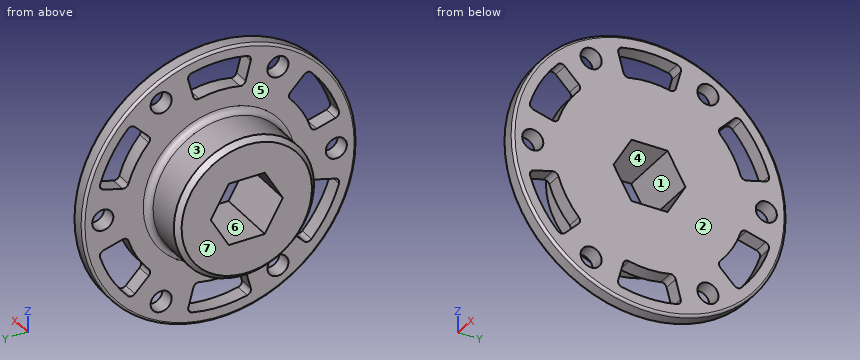
from build123d import *

# Parameters (mm, degrees)
SKETCH1_W                      = 3.175
SKETCH1_H                      = 27.94
CUT_EXTRUDE1_DEPTH             = 4.175
CUT_EXTRUDE2_DEPTH             = 4.175
CUT_EXTRUDE3_DEPTH             = 4.175
CUT_EXTRUDE4_DEPTH             = 4.175
CUT_EXTRUDE5_DEPTH             = 4.175
CUT_EXTRUDE6_DEPTH             = 4.175
SKETCH8_R                      = 14.294919975
BOSS_EXTRUDE1_DEPTH            = 9.525
CUT_EXTRUDE7_DEPTH             = 13.7
F_4_3_4_3_DIAMETER_HOLE1_D     = 4.3
F_4_3_4_3_DIAMETER_HOLE1_DEPTH = 12.7
CHAMFER1_SIZE                  = 1
FILLET1_R                      = 0.5
FILLET2_R                      = 1
FILLET3_R                      = 1.27


with BuildPart() as part:
    # Sketch1 → Revolve1 (revolve)
    with BuildSketch(Plane(origin=(0, 0, 0), x_dir=(-1, 0, 0), z_dir=(0, 0, -1))):
        with Locations((-11.1125, 13.97)):
            Rectangle(SKETCH1_W, SKETCH1_H)
    revolve(axis=Axis((12.7, 0, 0), (-1, 0, 0)))

    # Sketch2 → Cut-Extrude1 (cut, through all)
    with BuildSketch(Plane.ZY.offset(-9.525)):
        with BuildLine():
            Line((-13.806531048, -13.770610024), (-18.049174487, -18.013253463))
            ThreePointArc((-18.049174487, -18.013253463), (-12.738999884, -22.089995065), (-6.550803522, -24.644207701))
            Line((-6.550803522, -24.644207701), (-4.997885221, -18.848637704))
            ThreePointArc((-4.997885221, -18.848637704), (-9.738999389, -16.893841804), (-13.806531048, -13.770610024))
        make_face()
    extrude(amount=-CUT_EXTRUDE1_DEPTH, mode=Mode.SUBTRACT)

    # Sketch3 → Cut-Extrude2 (cut, through all)
    with BuildSketch(Plane.ZY.offset(-9.525)):
        with BuildLine():
            Line((5.022432582, -18.842111637), (6.57534786, -24.637670355))
            ThreePointArc((6.57534786, -24.637670355), (12.760996954, -22.077295051), (18.067108165, -17.995266116))
            Line((18.067108165, -17.995266116), (13.824456468, -13.752614419))
            ThreePointArc((13.824456468, -13.752614419), (9.760996476, -16.88114178), (5.022432582, -18.842111637))
        make_face()
    extrude(amount=-CUT_EXTRUDE2_DEPTH, mode=Mode.SUBTRACT)

    # Sketch4 → Cut-Extrude3 (cut, through all)
    with BuildSketch(Plane.ZY.offset(-9.525)):
        with BuildLine():
            Line((18.82896363, -5.071501614), (24.624522347, -6.624416892))
            ThreePointArc((24.624522347, -6.624416892), (25.499996837, 0.012700014), (24.617911686, 6.648941586))
            Line((24.617911686, 6.648941586), (18.822341689, 5.096023285))
            ThreePointArc((18.822341689, 5.096023285), (19.499995864, 0.012700024), (18.82896363, -5.071501614))
        make_face()
    extrude(amount=-CUT_EXTRUDE3_DEPTH, mode=Mode.SUBTRACT)

    # Sketch5 → Cut-Extrude4 (cut, through all)
    with BuildSketch(Plane.ZY.offset(-9.525)):
        with BuildLine():
            Line((13.806531048, 13.770610024), (18.049174487, 18.013253463))
            ThreePointArc((18.049174487, 18.013253463), (12.738999884, 22.089995065), (6.550803522, 24.644207701))
            Line((6.550803522, 24.644207701), (4.997885221, 18.848637704))
            ThreePointArc((4.997885221, 18.848637704), (9.738999389, 16.893841804), (13.806531048, 13.770610024))
        make_face()
    extrude(amount=-CUT_EXTRUDE4_DEPTH, mode=Mode.SUBTRACT)

    # Sketch6 → Cut-Extrude5 (cut, through all)
    with BuildSketch(Plane.ZY.offset(-9.525)):
        with BuildLine():
            Line((-24.617911686, -6.648941586), (-18.822341689, -5.096023285))
            ThreePointArc((-18.822341689, -5.096023285), (-19.499995864, -0.012700024), (-18.82896363, 5.071501614))
            Line((-18.82896363, 5.071501614), (-24.624522347, 6.624416892))
            ThreePointArc((-24.624522347, 6.624416892), (-25.499996837, -0.012700014), (-24.617911686, -6.648941586))
        make_face()
    extrude(amount=-CUT_EXTRUDE5_DEPTH, mode=Mode.SUBTRACT)

    # Sketch7 → Cut-Extrude6 (cut, through all)
    with BuildSketch(Plane(origin=(12.7, 0, 0), x_dir=(0, 0, -1), z_dir=(1, 0, 0))):
        with BuildLine():
            Line((6.57534786, 24.637670355), (5.022432582, 18.842111637))
            ThreePointArc((5.022432582, 18.842111637), (9.760996476, 16.88114178), (13.824456468, 13.752614419))
            Line((13.824456468, 13.752614419), (18.067108165, 17.995266116))
            ThreePointArc((18.067108165, 17.995266116), (12.760996954, 22.077295051), (6.57534786, 24.637670355))
        make_face()
    extrude(amount=-CUT_EXTRUDE6_DEPTH, mode=Mode.SUBTRACT)

    # Sketch8 → Boss-Extrude1 (add)
    with BuildSketch(Plane.ZY.offset(-9.525)):
        Circle(SKETCH8_R)
    extrude(amount=BOSS_EXTRUDE1_DEPTH)

    # Sketch9 → Cut-Extrude7 (cut, through all)
    with BuildSketch(Plane(origin=(12.7, 0, 0), x_dir=(0, 0, -1), z_dir=(1, 0, 0))):
        Polygon((-6.3627, 3.673506558), (-6.3627, -3.673506558), (0, -7.347013116), (6.3627, -3.673506558), (6.3627, 3.673506558), (0, 7.347013116), align=None)
    extrude(amount=-CUT_EXTRUDE7_DEPTH, mode=Mode.SUBTRACT)

    # Ø4.3 (4.3) Diameter Hole1
    with Locations(Plane(origin=(12.7, 0, 0), x_dir=(0, 0, -1), z_dir=(1, 0, 0))):
        with Locations((20.622229928, 11.90625), (20.622229928, -11.90625), (0, -23.8125), (-20.622229928, -11.90625), (-20.622229928, 11.90625), (0, 23.8125)):
            Hole(F_4_3_4_3_DIAMETER_HOLE1_D / 2, depth=F_4_3_4_3_DIAMETER_HOLE1_DEPTH)

    # Chamfer1
    chamfer1_edges = [part.edges().sort_by_distance(p)[0] for p in [
        (0, 0, -14.294919975),
    ]]
    chamfer(chamfer1_edges, length=CHAMFER1_SIZE)

    # Fillet1
    fillet1_edges = [part.edges().sort_by_distance(p)[0] for p in [
        (9.525, -27.94, 0),
        (12.7, -27.94, 0),
    ]]
    fillet(fillet1_edges, radius=FILLET1_R)

    # Fillet2
    fillet2_edges = [part.edges().sort_by_distance(p)[0] for p in [
        (11.1125, -13.770610024, -13.806531048),
        (11.1125, -18.848637704, -4.997885221),
        (11.1125, -24.644207701, -6.550803522),
        (11.1125, -18.013253463, -18.049174487),
        (11.1125, -18.842111637, 5.022432582),
        (11.1125, -13.752614419, 13.824456468),
        (11.1125, -17.995266116, 18.067108165),
        (11.1125, -24.637670355, 6.57534786),
        (11.1125, -5.071501614, 18.82896363),
        (11.1125, 5.096023285, 18.822341689),
        (11.1125, 6.648941586, 24.617911686),
        (11.1125, -6.624416892, 24.624522347),
        (11.1125, 13.770610024, 13.806531048),
        (11.1125, 18.848637704, 4.997885221),
        (11.1125, 24.644207701, 6.550803522),
        (11.1125, 18.013253463, 18.049174487),
        (11.1125, -6.648941586, -24.617911686),
        (11.1125, 6.624416892, -24.624522347),
        (11.1125, 5.071501614, -18.82896363),
        (11.1125, -5.096023285, -18.822341689),
        (11.1125, 24.637670355, -6.57534786),
        (11.1125, 17.995266116, -18.067108165),
        (11.1125, 13.752614419, -13.824456468),
        (11.1125, 18.842111637, -5.022432582),
    ]]
    fillet(fillet2_edges, radius=FILLET2_R)

    # Fillet3
    fillet3_edges = [part.edges().sort_by_distance(p)[0] for p in [
        (9.525, 0, -14.294919975),
    ]]
    fillet(fillet3_edges, radius=FILLET3_R)


solid = part.part
The model under review builds one solid part; all positions refer to its coordinate system, in mm. Face numbers are marked on the shaded views. A direction names the side the tool comes from. Give positions to 0.01 mm unless a question says otherwise; leave off trailing zeros. Write each loop counter-clockwise with the first axis right and the second up, starting at its lowest first coordinate (ties: lowest second). Pieces come first, ordered by that corner, then holes.
1. Wall thickness on L1, parallel to Y at x = 11.25, z = 0; L2, parallel to Z at x = 10.5, y = 21; L3, parallel to Y at x = 4.5, z = -13: over which ranges is each line inside the solid? List them lowest first.
2. Add section B-B, the plane x = 5.25. Write out the cut boundary in (y, z), plus the area to 3 significant figures.
3. Add section A-A, the plane y = 0. Write out the cut boundary in (x, z) (3 decimals).
4. Draft analysis for pull direction Y (two halves, no side actions). For the marked faces 1, 2, 3 and 4, state which applies: +Y half, -Y half, draft (parallel to the pull), parting line (faces both ways), or undercut.
5. Tool access review of the marked faces 5, 6 and 7: name each direction out of +Z, -Z, +X, -X, +Y, -Y from which nothing blocks a thin tool from reaching the whole face with its end or side.
6. Add section C-C, the plane z = -10. Count the separate pieces of the cut face and the enclosed holes in it, plus the area to 3 significant figures.
7. For P1, Ø6, axis at x = 7.5, z = 9, coming from the -Y side; P2, Ø7, axis at y = 11.91, z = 20.62, coming from the -X side (3 decimals); P3, Ø5, axis at x = 9.5, y = -2, coming from the -Z side; P4, Ø5.5, axis at y = 23.81, z = 0, coming from the +X side, all flat-tipped, find the tip position at first contact; note any pin that passes through.
Worked answers:
1. L1: y = -27.94 to -25.96, -21.66 to -7.35, 7.35 to 21.66, 25.96 to 27.94
1. L2: z = -18.43 to -14.47, -5.6 to 5.57, 14.47 to 18.43
1. L3: y = -5.95 to 5.95
2. outline: circle Ø28.59 at (0, 0); hole (-7.35, 0) - (-3.67, -6.36) - (3.67, -6.36) - (7.35, 0) - (3.67, 6.36) - (-3.67, 6.36) - close
2. area: 502 mm2
3. outline: (0, -13.295) - (1, -14.295) - (8.255, -14.295) arc R1.27 cw to (9.525, -15.565) - (9.525, -19.5) - (12.7, -19.5) - (12.7, -6.363) - (0, -6.363) - close; (0, 6.363) - (12.7, 6.363) - (12.7, 19.5) - (9.525, 19.5) - (9.525, 15.565) arc R1.27 cw to (8.255, 14.295) - (1, 14.295) - (0, 13.295) - close; (9.525, -27.44) arc R0.5 ccw to (10.025, -27.94) - (12.2, -27.94) arc R0.5 ccw to (12.7, -27.44) - (12.7, -25.5) - (9.525, -25.5) - close; (9.525, 25.5) - (12.7, 25.5) - (12.7, 27.44) arc R0.5 ccw to (12.2, 27.94) - (10.025, 27.94) arc R0.5 ccw to (9.525, 27.44) - close
4. face 1: undercut
4. face 2: draft
4. face 3: parting line
4. face 4: undercut
5. face 5: -X
5. face 6: +X, -X
5. face 7: +Z, -Z, -X, +Y, -Y
6. separate pieces: 3
6. enclosed holes: 0
6. area: 317 mm2
7. P1: stops at y = -26.98
7. P2: stops at x = 9.525
7. P3: stops at z = -27.94
7. P4: stops at x = 12.7
